Verification items for the finished model (mm, model axes). A direction names the side the tool comes from. Round coordinates to 2 decimals unless told otherwise and drop trailing zeros. Order: outer loops, then holes, each group sorted by start corner. A loop starts at its lowest first (then second) coordinate and runs counter-clockwise, first axis right, second up. Notation, with made-up numbers: M -27,-13 L 0,-13 A33 ccw 0,21 Z; hole C 46.25,53.25 d5. An arc over 180 degrees is marked long. Use one line per item in the form item = value. Start each with the question number.
Item 1: Go/stop test with flat-tipped pins: pin 1 Ø3 at (x, z) = (37.5, 10) entering from -Y; pin 2 Ø0.8 at (y, z) = (-0.5, 20.5) entering from +X; pin 3 Ø3 at (y, z) = (-23.5, 12) entering from -X; pin 4 Ø1.3 at (x, z) = (30, 5.5) entering from -Y. Record where each tip stops, or that it passes through.
Item 2: Thickness scan on probe 1 along Z at (x, y) = (5, -1.95); probe 2 along Y at (x, z) = (40, 29); probe 3 along X at (y, z) = (-26, 34). Record the ranges inside material, lowest first. Write a range as [from, to].
Item 3: Release check for a two-part mould opening along X. For faces 6 (the cylindrical face through (25.1, -2.01, 30.14)), 7 (the flat face through (66, -36, 18)), 8 (the flat face through (67, -20, 18)) record: +X half, -X half, draft (parallel to the pull), parting line (faces both ways), or undercut.
Item 4: Cross-section at C-C on z = 14.5. Enter the section's corners in (x, y).
Item 5: Cross-section at D-D on x = 25. Enter the section's corners in (y, z).
Item 6: Cross-section at B-B on y = -12. Enter the section's corners in (x, z), then the cut area to 3 significant figures.
Item 7: Cross-section at A-A on z = 26. Enter the section's corners in (x, y), then the cut area to 3 significant figures.
Item 8: Tool access check on faces 1 (the cylindrical face through (0.86, -1.48, 35.1)), 2 (the flat face through (65, -20, 24.4)), 3 (the flat face through (38, -3, 18)), 4 (the cylindrical face through (9.9, -2.01, 5.86)), 5 (the flat face through (6, -1, 14)). Record the directions out of +Z, -Z, +X, -X, +Y, -Y that give a thin tool (end or side, any length) a straight path to the whole face; none if there is none.
from build123d import *

# Parameters (mm, degrees)
EXTRUDE_1_DEPTH     = 36
SKETCH_2_R          = 1.1
SKETCH_2_W          = 17
SKETCH_2_H          = 26
CUT_EXTRUDE_1_DEPTH = 12
SKETCH_3_R          = 1.6
CUT_EXTRUDE_2_DEPTH = 22
FILLET_1_R          = 3
CUT_EXTRUDE_3_DEPTH = 1


with BuildPart() as part:
    # 草图1 → 凸台-拉伸1 (new body)
    with BuildSketch(Plane.XY):
        Polygon((0, 0), (67, 0), (67, -2), (67, -36), (64, -36), (64, -3), (0, -3), align=None)
    extrude(amount=EXTRUDE_1_DEPTH)

    # 草图2 → 切除-拉伸1 (cut)
    with BuildSketch(Plane(origin=(0, 0, 0), x_dir=(1, 0, 0), z_dir=(0, 1, 0))):
        with Locations(Location((5, -5.5, 0), (0, 0, 270))):
            Circle(SKETCH_2_R)
        with Locations(Location((5, -29.5, 0), (0, 0, 270))):
            Circle(SKETCH_2_R)
        with Locations(Location((30, -5.5, 0), (0, 0, 270))):
            Circle(SKETCH_2_R)
        with Locations(Location((30, -29.5, 0), (0, 0, 270))):
            Circle(SKETCH_2_R)
        with Locations((17.5, -18)):
            Rectangle(SKETCH_2_W, SKETCH_2_H)
    extrude(amount=-CUT_EXTRUDE_1_DEPTH, mode=Mode.SUBTRACT)

    # 草图3 → 切除-拉伸2 (cut)
    with BuildSketch(Plane.ZY.offset(-64)):
        with Locations(Location((7, -27.215224582, 0), (0, 0, 270))):
            Circle(SKETCH_3_R)
        with BuildLine():
            Line((27.6, -10), (27.6, -29))
            ThreePointArc((27.6, -29), (26, -30.6), (24.4, -29))
            Line((24.4, -29), (24.4, -10))
            ThreePointArc((24.4, -10), (26, -8.4), (27.6, -10))
        make_face()
    extrude(amount=-CUT_EXTRUDE_2_DEPTH, mode=Mode.SUBTRACT)

    # 圆角1
    fillet_1_edges = [part.edges().sort_by_distance(p)[0] for p in [
        (0, -1.5, 0),
        (67, 0, 18),
        (64, -3, 18),
        (9, -1.5, 31),
        (9, -1.5, 5),
        (26, -1.5, 5),
        (26, -1.5, 31),
        (0, -1.5, 36),
    ]]
    fillet(fillet_1_edges, radius=FILLET_1_R)

    # 草图4 → 切除-拉伸3 (cut)
    with BuildSketch(Plane(origin=(0, 0, 0), x_dir=(1, 0, 0), z_dir=(0, 1, 0))):
        Polygon((5, -4.4), (5, -30.6), (5, -32.6), (30, -32.6), (30, -30.6), (30, -4.4), (30, -2.4), (5, -2.4), align=None)
    extrude(amount=-CUT_EXTRUDE_3_DEPTH, mode=Mode.SUBTRACT)


solid = part.part
Output values:
q1.pin_1 = -3
q1.pin_2 = 66.14
q1.pin_3 = 64
q1.pin_4 = through
q2.probe_1 = [0, 4.4], [6.6, 28.4], [30.6, 36]
q2.probe_2 = [-3, 0]
q2.probe_3 = [64, 67]
q3.face_6 = undercut
q3.face_7 = draft
q3.face_8 = +X half
q4.outline = M 0,-3 L 9,-3 L 9,-1 L 5,-1 L 5,0 L 0,0 Z; M 26,-3 L 61,-3 A3 cw 64,-6 L 64,-36 L 67,-36 L 67,-3 A3 ccw 64,0 L 30,0 L 30,-1 L 26,-1 Z
q5.outline = M -3,0 L 0,0 L 0,2.4 L -1,2.4 L -1,5.76 L -3,5.76 Z; M -3,30.24 L -1,30.24 L -1,32.6 L 0,32.6 L 0,36 L -3,36 Z
q6.outline = M 64,0 L 67,0 L 67,24.4 L 64,24.4 Z; M 64,27.6 L 67,27.6 L 67,36 L 64,36 Z
q6.area = 98.4 mm2
q7.outline = M 0,-3 L 9,-3 L 9,-1 L 5,-1 L 5,0 L 0,0 Z; M 26,-3 L 61,-3 A3 cw 64,-6 L 64,-8.4 L 67,-8.4 L 67,-3 A3 ccw 64,0 L 30,0 L 30,-1 L 26,-1 Z; M 64,-36 L 67,-36 L 67,-30.6 L 64,-30.6 Z
q7.area = 174 mm2
q8.face_1 = +Z, -X, +Y, -Y
q8.face_2 = +X, -X
q8.face_3 = +Z, -Z, -X, -Y
q8.face_4 = +Y, -Y
q8.face_5 = +Y
